Drawing for the job (mm, zero at the part's lowest x, y, z). A direction names the side the tool comes from. Give positions to 0.01 mm unless a question says otherwise; leave off trailing zeros. Loops run counter-clockwise (first coordinate to the right, second up) from the corner with the lowest first, then second, coordinate; pieces in that order, holes last. Notation, with made-up numbers: (-6, 22.5) -> (45, 22.5) arc R22 ccw to (45, 52.5) -> close; hole circle Ø8 at (51.5, 59.5). An arc over 180 degrees is marked (long way). Use CSV: the item, a comma, the result in double quotes. Start each with the question number.
(1) 3-axis set-ups, long thin cutter, end or side, ignore diameter. For the marked faces 1, 2 and 3: which of +Z, -Z, +X, -X, +Y, -Y reach the whole face in a straight line?
(2) Cut at C-C on y = 10.5. Write the cut outline in (x, z) (1 decimal), then the cut area to 3 significant figures.
(3) Flat gauge pins, fed straight in: pin 1 (7 mm diameter, centred on x = 11, z = 13.5, fed in from -Y); pin 2 (8 mm diameter, centred on y = 5.5, z = 12.5, fed in from -X); pin 3 (1 mm diameter, centred on y = 4.5, z = 3.5, fed in from -X); pin 4 (7 mm diameter, centred on x = 14.5, y = 20.5, fed in from +Z). Where does each tip first touch, or does it go through?
(4) Cut at D-D on z = 2.75. Write the cut outline in (x, y).
(5) Drill centre lines: probe 1 along Y at (x, z) = (3.25, 19.5); probe 2 along Z at (x, y) = (4.5, 1.5); probe 3 along Z at (x, y) = (3.25, 9) (1 decimal). Where is each one in solid material? Low to high.
(6) Cut at B-B on x = 6. Write the cut outline in (y, z) (1 decimal), then the cut area to 3 significant figures.
(7) Cut at A-A on z = 17.75. Write the cut outline in (x, y), then the cut area to 3 significant figures.
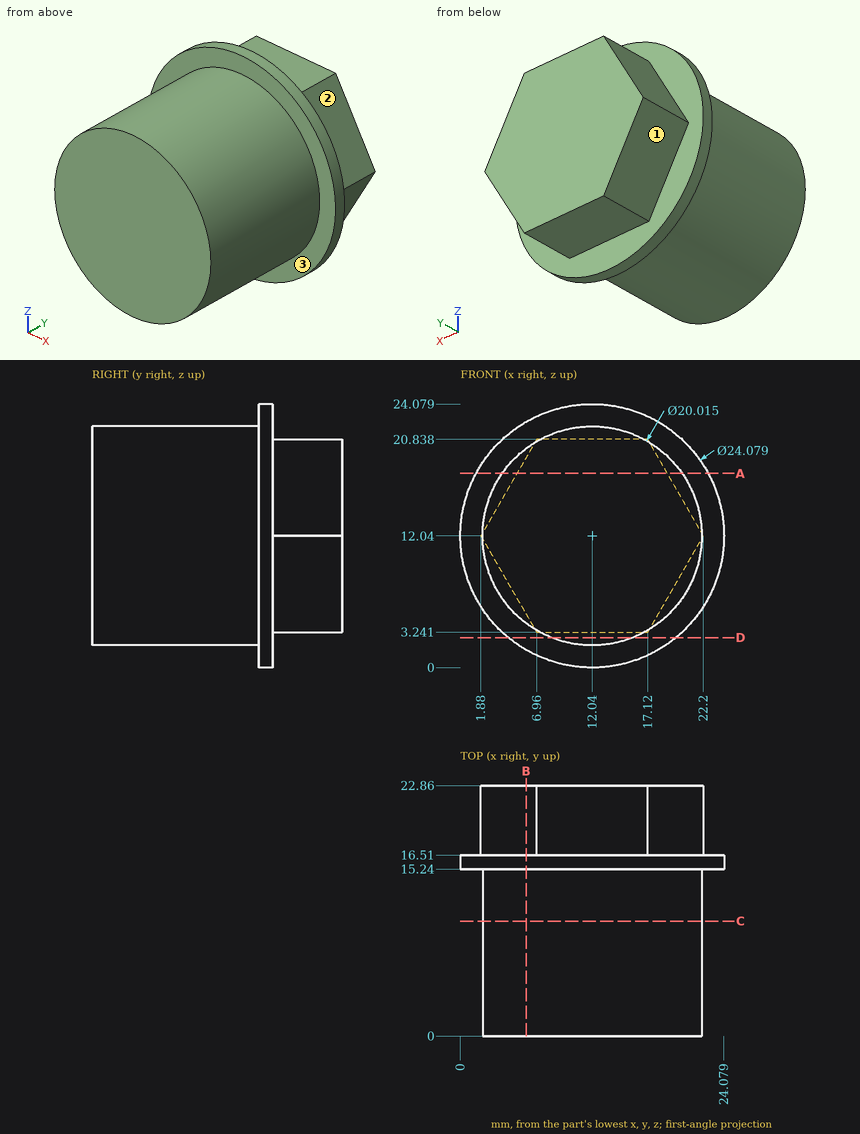
Check result:
1,face 1,"-Z, -X, +Y"
1,face 2,"+Z, +X, +Y"
1,face 3,"-Y"
2,outline,"circle Ø20 at (12, 12)"
2,area,"315 mm²"
3,pin 1,"y = 0"
3,pin 2,"x = 2.03"
3,pin 3,"x = 6.08"
3,pin 4,"z = 20.84"
4,outline,"(4.38, 15.24) -> (8.32, 15.24) -> (8.32, 0) -> (15.76, 0) -> (15.76, 15.24) -> (19.7, 15.24) -> (19.7, 16.51) -> (4.38, 16.51) -> close"
5,probe 1,"15.24 to 16.51"
5,probe 2,"5.46 to 18.62"
5,probe 3,"7.3 to 16.8"
6,outline,"(0, 4.1) -> (15.2, 4.1) -> (15.2, 1.6) -> (16.5, 1.6) -> (16.5, 4.9) -> (22.9, 4.9) -> (22.9, 19.2) -> (16.5, 19.2) -> (16.5, 22.5) -> (15.2, 22.5) -> (15.2, 20) -> (0, 20) -> close"
6,area,"360 mm²"
7,outline,"(1.44, 15.24) -> (3.82, 15.24) -> (3.82, 0) -> (20.26, 0) -> (20.26, 15.24) -> (22.64, 15.24) -> (22.64, 16.51) -> (18.9, 16.51) -> (18.9, 22.86) -> (5.18, 22.86) -> (5.18, 16.51) -> (1.44, 16.51) -> close"
7,area,"365 mm²"
